Geometry check sheet. Reference: the model listing, model coordinates, mm. Face numbers are marked on the shaded views. A direction names the side the tool comes from. Give positions to 0.01 mm unless a question says otherwise; leave off trailing zeros. Use a Markdown table: item, result. Add a question column.
1. Depth check by flat-ended pin: P1, Ø2, axis at x = 10, z = 3.5, coming from the -Y side; P2, Ø6, axis at x = -4, z = 1.5, coming from the +Y side; P3, Ø5, axis at y = -11, z = 5.5, coming from the +X side; P4, Ø1.5, axis at y = 0.5, z = 1, coming from the +X side. Enter the tip coordinate at first touch or a pass-through.
2. Material ranges on L1, parallel to Y at x = -15.5, z = 6; L2, parallel to X at y = -16, z = 6; L3, parallel to X at y = -10, z = 5.5, recorded low to high.
3. Set-up check for the marked faces 4, 5, 6 and 7: record each of +Z, -Z, +X, -X, +Y, -Y from which the full face is reachable in a straight line by a thin tool's end or side.
4. Draft check along X on the marked faces 1, 2 and 3. Enter one of: pulls with the +X half, pulls with the -X half, needs draft (parallel to the pull), parting line crosses it, or undercut.
from build123d import *

# Parameters (mm, degrees)
F1_DEPTH = 10


with BuildPart() as f1:
    # F0 (on Top) → F1 (new body)
    with BuildSketch(Plane.XY):
        with BuildLine():
            ThreePointArc((0.834247, 13.754724), (0.539473, 13.922611), (0.384061, 14.224148))
            ThreePointArc((0.384061, 14.224148), (-0.053041, 16.126356), (-1.146638, 17.742988))
            Line((-1.146638, 17.742988), (-1.950006, 17.672744))
            ThreePointArc((-1.950006, 17.672744), (-2.74627, 15.891587), (-2.846993, 13.943148))
            ThreePointArc((-2.846993, 13.943148), (-2.94723, 13.618388), (-3.20868, 13.401223))
            Line((-3.20868, 13.401223), (-3.920457, 13.210542))
            ThreePointArc((-3.920457, 13.210542), (-4.254874, 13.267486), (-4.504046, 13.497684))
            ThreePointArc((-4.504046, 13.497684), (-5.565381, 15.135677), (-7.145946, 16.280782))
            Line((-7.145946, 16.280782), (-7.876841, 15.940006))
            ThreePointArc((-7.876841, 15.940006), (-8.015892, 13.993927), (-7.444136, 12.128545))
            ThreePointArc((-7.444136, 12.128545), (-7.427254, 11.789086), (-7.598661, 11.495597))
            Line((-7.598661, 11.495597), (-8.202296, 11.072974))
            ThreePointArc((-8.202296, 11.072974), (-8.536021, 11.012106), (-8.848898, 11.1432))
            ThreePointArc((-8.848898, 11.1432), (-10.406453, 12.319412), (-12.283348, 12.854873))
            Line((-12.283348, 12.854873), (-12.853612, 12.284668))
            ThreePointArc((-12.853612, 12.284668), (-12.31868, 10.408393), (-11.143406, 8.85106))
            ThreePointArc((-11.143406, 8.85106), (-11.01144, 8.537847), (-11.072132, 8.203432))
            Line((-11.072132, 8.203432), (-11.494817, 7.599841))
            ThreePointArc((-11.494817, 7.599841), (-11.787598, 7.428503), (-12.126443, 7.444681))
            ThreePointArc((-12.126443, 7.444681), (-13.992354, 8.017243), (-15.939197, 7.878477))
            Line((-15.939197, 7.878477), (-16.280048, 7.147617))
            ThreePointArc((-16.280048, 7.147617), (-15.135653, 5.567454), (-13.498617, 4.506006))
            ThreePointArc((-13.498617, 4.506006), (-13.267485, 4.256818), (-13.21014, 3.921813))
            Line((-13.21014, 3.921813), (-13.400893, 3.210056))
            ThreePointArc((-13.400893, 3.210056), (-13.617417, 2.948914), (-13.94136, 2.848224))
            ThreePointArc((-13.94136, 2.848224), (-15.890571, 2.748077), (-17.672544, 1.95182))
            Line((-17.672544, 1.95182), (-17.74287, 1.148459))
            ThreePointArc((-17.74287, 1.148459), (-16.127043, 0.054997), (-14.225696, -0.382538))
            ThreePointArc((-14.225696, -0.382538), (-13.923275, -0.537647), (-13.75481, -0.832836))
            Line((-13.75481, -0.832836), (-13.690624, -1.566909))
            ThreePointArc((-13.690624, -1.566909), (-13.804774, -1.886358), (-14.074743, -2.091771))
            ThreePointArc((-14.074743, -2.091771), (-15.87215, -2.852547), (-17.274321, -4.210255))
            Line((-17.274321, -4.210255), (-17.06564, -4.989221))
            ThreePointArc((-17.06564, -4.989221), (-15.173273, -5.464093), (-13.236946, -5.224943))
            ThreePointArc((-13.236946, -5.224943), (-12.899713, -5.267264), (-12.640446, -5.487031))
            Line((-12.640446, -5.487031), (-12.329064, -6.154883))
            ThreePointArc((-12.329064, -6.154883), (-12.327072, -6.494108), (-12.510505, -6.779467))
            ThreePointArc((-12.510505, -6.779467), (-13.939314, -8.109113), (-14.79256, -9.864511))
            Line((-14.79256, -9.864511), (-14.330042, -10.525127))
            ThreePointArc((-14.330042, -10.525127), (-12.389383, -10.324133), (-10.651624, -9.437142))
            ThreePointArc((-10.651624, -9.437142), (-10.320255, -9.36157), (-10.001459, -9.47941))
            Line((-10.001459, -9.47941), (-9.480437, -10.000486))
            ThreePointArc((-9.480437, -10.000486), (-9.362542, -10.318572), (-9.437314, -10.64946))
            ThreePointArc((-9.437314, -10.64946), (-10.32519, -12.387599), (-10.526598, -14.328962))
            Line((-10.526598, -14.328962), (-9.86603, -14.791547))
            ThreePointArc((-9.86603, -14.791547), (-8.11115, -13.93893), (-6.78156, -12.511083))
            ThreePointArc((-6.78156, -12.511083), (-6.496022, -12.326734), (-6.156148, -12.328432))
            Line((-6.156148, -12.328432), (-5.488329, -12.639883))
            ThreePointArc((-5.488329, -12.639883), (-5.268753, -12.898464), (-5.225845, -13.234971))
            ThreePointArc((-5.225845, -13.234971), (-5.465697, -15.171959), (-4.990972, -17.065128))
            Line((-4.990972, -17.065128), (-4.212028, -17.273888))
            ThreePointArc((-4.212028, -17.273888), (-2.854593, -15.872486), (-2.093539, -14.076003))
            ThreePointArc((-2.093539, -14.076003), (-1.888272, -13.805111), (-1.568315, -13.690463))
            Line((-1.568315, -13.690463), (-0.834247, -13.754724))
            ThreePointArc((-0.834247, -13.754724), (-0.539473, -13.922611), (-0.384061, -14.224148))
            ThreePointArc((-0.384061, -14.224148), (0.053041, -16.126356), (1.146638, -17.742988))
            Line((1.146638, -17.742988), (1.950006, -17.672744))
            ThreePointArc((1.950006, -17.672744), (2.74627, -15.891587), (2.846993, -13.943148))
            ThreePointArc((2.846993, -13.943148), (2.94723, -13.618388), (3.20868, -13.401223))
            Line((3.20868, -13.401223), (3.920457, -13.210542))
            ThreePointArc((3.920457, -13.210542), (4.254874, -13.267486), (4.504046, -13.497684))
            ThreePointArc((4.504046, -13.497684), (5.565381, -15.135677), (7.145946, -16.280782))
            Line((7.145946, -16.280782), (7.876841, -15.940006))
            ThreePointArc((7.876841, -15.940006), (8.015892, -13.993927), (7.444136, -12.128545))
            ThreePointArc((7.444136, -12.128545), (7.427254, -11.789086), (7.598661, -11.495597))
            Line((7.598661, -11.495597), (8.202296, -11.072974))
            ThreePointArc((8.202296, -11.072974), (8.536021, -11.012106), (8.848898, -11.1432))
            ThreePointArc((8.848898, -11.1432), (10.406453, -12.319412), (12.283348, -12.854873))
            Line((12.283348, -12.854873), (12.853612, -12.284668))
            ThreePointArc((12.853612, -12.284668), (12.31868, -10.408393), (11.143406, -8.85106))
            ThreePointArc((11.143406, -8.85106), (11.01144, -8.537847), (11.072132, -8.203432))
            Line((11.072132, -8.203432), (11.494817, -7.599841))
            ThreePointArc((11.494817, -7.599841), (11.787598, -7.428503), (12.126443, -7.444681))
            ThreePointArc((12.126443, -7.444681), (13.992354, -8.017243), (15.939197, -7.878477))
            Line((15.939197, -7.878477), (16.280048, -7.147617))
            ThreePointArc((16.280048, -7.147617), (15.135653, -5.567454), (13.498617, -4.506006))
            ThreePointArc((13.498617, -4.506006), (13.267485, -4.256818), (13.21014, -3.921813))
            Line((13.21014, -3.921813), (13.400893, -3.210056))
            ThreePointArc((13.400893, -3.210056), (13.617417, -2.948914), (13.94136, -2.848224))
            ThreePointArc((13.94136, -2.848224), (15.890571, -2.748077), (17.672544, -1.95182))
            Line((17.672544, -1.95182), (17.74287, -1.148459))
            ThreePointArc((17.74287, -1.148459), (16.127043, -0.054997), (14.225696, 0.382538))
            ThreePointArc((14.225696, 0.382538), (13.923275, 0.537647), (13.75481, 0.832836))
            Line((13.75481, 0.832836), (13.690624, 1.566909))
            ThreePointArc((13.690624, 1.566909), (13.804774, 1.886358), (14.074743, 2.091771))
            ThreePointArc((14.074743, 2.091771), (15.87215, 2.852547), (17.274321, 4.210255))
            Line((17.274321, 4.210255), (17.06564, 4.989221))
            ThreePointArc((17.06564, 4.989221), (15.173273, 5.464093), (13.236946, 5.224943))
            ThreePointArc((13.236946, 5.224943), (12.899713, 5.267264), (12.640446, 5.487031))
            Line((12.640446, 5.487031), (12.329064, 6.154883))
            ThreePointArc((12.329064, 6.154883), (12.327072, 6.494108), (12.510505, 6.779467))
            ThreePointArc((12.510505, 6.779467), (13.939314, 8.109113), (14.79256, 9.864511))
            Line((14.79256, 9.864511), (14.330042, 10.525127))
            ThreePointArc((14.330042, 10.525127), (12.389383, 10.324133), (10.651624, 9.437142))
            ThreePointArc((10.651624, 9.437142), (10.320255, 9.36157), (10.001459, 9.47941))
            Line((10.001459, 9.47941), (9.480437, 10.000486))
            ThreePointArc((9.480437, 10.000486), (9.362542, 10.318572), (9.437314, 10.64946))
            ThreePointArc((9.437314, 10.64946), (10.32519, 12.387599), (10.526598, 14.328962))
            Line((10.526598, 14.328962), (9.86603, 14.791547))
            ThreePointArc((9.86603, 14.791547), (8.11115, 13.93893), (6.78156, 12.511083))
            ThreePointArc((6.78156, 12.511083), (6.496022, 12.326734), (6.156148, 12.328432))
            Line((6.156148, 12.328432), (5.488329, 12.639883))
            ThreePointArc((5.488329, 12.639883), (5.268753, 12.898464), (5.225845, 13.234971))
            ThreePointArc((5.225845, 13.234971), (5.465697, 15.171959), (4.990972, 17.065128))
            Line((4.990972, 17.065128), (4.212028, 17.273888))
            ThreePointArc((4.212028, 17.273888), (2.854593, 15.872486), (2.093539, 14.076003))
            ThreePointArc((2.093539, 14.076003), (1.888272, 13.805111), (1.568315, 13.690463))
            Line((1.568315, 13.690463), (0.834247, 13.754724))
        make_face()
        Polygon((0, 5.1), (4.850388, 1.575987), (2.997705, -4.125987), (-2.997705, -4.125987), (-4.850388, 1.575987), align=None, mode=Mode.SUBTRACT)
    extrude(amount=F1_DEPTH)


solid = f1.part
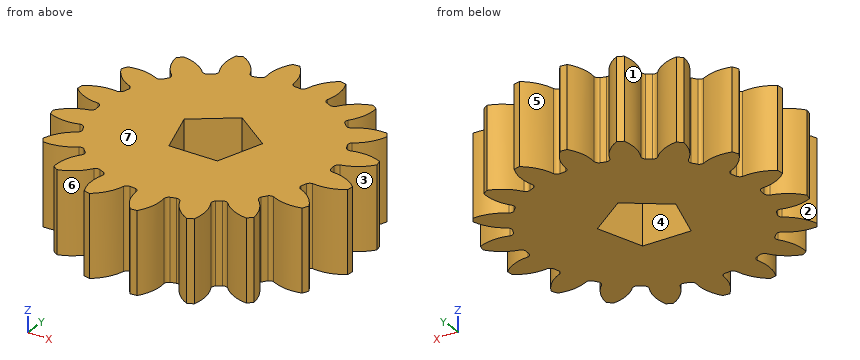
Values found:
| question | item | result |
|---|---|---|
| 1 | P1 | stops at y = -12.57 |
| 1 | P2 | stops at y = 17.74 |
| 1 | P3 | stops at x = 12.85 |
| 1 | P4 | stops at x = 16.53 |
| 2 | L1 | y = -5.43 to -2.63, -0.17 to 2.83, 5.95 to 7.97 |
| 2 | L2 | x = -5.35 to -2.94, 0 to 2.72, 6.63 to 7.75 |
| 2 | L3 | x = -14.7 to -11.56, -9.48 to 12.09 |
| 3 | face 4 | +Z, -Z |
| 3 | face 5 | +Z, -Z, +Y |
| 3 | face 6 | +Z, -Z, -Y |
| 3 | face 7 | +Z, +X, -X, +Y, -Y |
| 4 | face 1 | undercut |
| 4 | face 2 | pulls with the -X half |
| 4 | face 3 | pulls with the +X half |
